Model file for the job. Use its own axes, mm. A direction names the side the tool comes from. Coordinates: 2 decimals unless noted, no trailing zeros. Loops run counter-clockwise (first coordinate to the right, second up) from the corner with the lowest first, then second, coordinate; pieces in that order, holes last. Notation, with made-up numbers: M 46.5,26 L 85.5,26 A25 ccw 85.5,63 Z; hole C 77,-11.75 d1. An arc over 180 degrees is marked long. Write item = value, one per line. Start each with the question number.
Autodesk Inventor part; units mm, degrees
ref_plane "YZ Plane" through (0, 0, 0) normal (1, 0, 0) x (0, 1, 0)
ref_plane "XZ Plane" through (0, 0, 0) normal (0, 1, 0) x (-1, 0, 0)
ref_plane "XY Plane" through (0, 0, 0) normal (0, 0, 1) x (1, 0, 0)
sketch "Sketch1" plane through (0, 0, 0) normal (0, 1, 0) x (-1, 0, 0)
  line L0 (0, 0) -> (108.6, 0)
  line L1 (108.6, 0) -> (108.6, -110.4)
  line L2 (108.6, -110.4) -> (0, -110.4)
  line L3 (0, -110.4) -> (0, 0)
  circle A0 centre (12.3, -77.7) radius 6.5
  circle A1 centre (57.3, -77.7) radius 12
  dimension "d0" = 108.6
  dimension "d1" = 110.4
  dimension "d2" = 13
  dimension "altura_hoyo" = 12.3
  dimension "d5" = 32.7
  dimension "d6" = 24
  dimension "d7" = 45
extrude "Extrusion1" add sketch "Sketch1" along normal blind 27
sketch "Sketch2" plane through (0, 27, 0) normal (0, 1, 0) x (1, 0, 0)
  line L0 (0, 110.4) -> (-108.6, 110.4) construction
  line L1 (0, 0) -> (0, -195.629)
  line L2 (0, -195.629) -> (0, -201.129)
  line L3 (0, -201.129) -> (-188.5967, -306.4251)
  line L4 (-24.6, 0) -> (-24.6, -190.129)
  line L5 (-188.5967, -281.6906) -> (-24.6, -190.129)
  line L6 (-188.5967, -306.4251) -> (-188.5967, -281.6906)
  circle A0 centre (-12.3, -195.629) radius 7.8
  circle A1 centre (-12.3, 77.7) radius 6.5 construction
  line L7 (-108.6, 0) -> (0, 0)
  line L8 (0, 0) -> (-24.6, 0)
  line L9 (-12.3, -195.629) -> (-149.732, -272.3592) construction
  line L10 (0, -201.129) -> (-12.3, -195.629) construction
  line L11 (-42.6296, -182.067) -> (-12.3, -195.629) construction
  circle A2 centre (-149.732, -272.3592) radius 7.8
  dimension "d10" = 306.029
  dimension "d11" = 5.5
  dimension "d12" = 119.175
  dimension "Ancho_marco" = 24.6
  dimension "d18" = 15.6
  dimension "d21" = 216
  dimension "d26" = 12.3
  dimension "d_entre_ejes" = 157.401
  dimension "d28" = 15.6
  dimension "d31" = 195.629
  dimension "d32" = 273.329
extrude "Extrusion2" add sketch "Sketch2" against normal blind 27 contours L1 L2 L3 L6 L5 L4 L7 | A2
fillet "Fillet1" radius 10 2 edges at (-24.6, 13.5, 190.129) (0, 13.5, 201.129)
sketch "Sketch3" plane through (0, 27, 0) normal (0, 1, 0) x (1, 0, 0)
  line L0 (-188.5967, -281.6906) -> (-188.5967, -306.4251)
  line L1 (-188.5967, -306.4251) -> (-200.2967, -306.4251)
  line L2 (-200.2967, -306.4251) -> (-200.2967, -288.2229)
  line L3 (-188.5967, -306.4251) -> (-188.5967, -281.6906)
  line L4 (-188.5967, -281.6906) -> (-200.2967, -288.2229)
  line L5 (-29.7252, -192.9905) -> (-188.5967, -281.6906)
  point P0 (0, 0)
  dimension "d23" = 11.7
extrude "Extrusion3" add sketch "Sketch3" against normal blind 27
extrude "Extrusion4" cut sketch "Sketch2" against normal blind 27 contours A2
equation "\"d11\" = 0.5 * D_eje"
equation "\"d18\" = d28"
properties part number "Marco_triciclo" material "Aluminum 6061"
Item 1: Probe L1, parallel to Z at x = -57.3, y = 9; L2, parallel to Z at x = -14.5, y = 3.25; L3, parallel to Z at x = -77, y = 22. List the from-to ranges inside material, lowest first.
Item 2: Cut at C-C (y = 16.25). Give the cut face in (x, z), plus the area to 3 significant figures.
Item 3: Pull direction X, two halves, no side cores. Call faces 4 (the flat face through (-95.577, 13.689, 254.491)), 5 (the cylindrical face through (-25.94, 13.31, 189.26)), 6 (the cylindrical face through (-68.746, 13.311, -81.304)): +X half, -X half, draft (parallel to the pull), parting line (faces both ways), or undercut.
Item 4: 3-axis set-ups, long thin cutter, end or side, ignore diameter. For faces 1 (the flat face through (-19, 0, 35)), 2 (the flat face through (-24.6, 14, 91)), 3 (the flat face through (-108.6, 13, -54)): which of +Z, -Z, +X, -X, +Y, -Y reach the whole face in a straight line?
Item 5: Cut at D-D (z = -11.5). Give the cut face in (x, y), plus the area to 3 significant figures.
Item 6: Pin check, flat tips, straight feed: pin 1 Ø8 at (y, z) = (16, 108.5) entering from -X; pin 2 Ø13.5 at (y, z) = (11.5, -29.5) entering from -X. Stop position of each tip, or through.
Item 7: Cut at A-A (z = -77.7). Give the cut face in (x, y), plus the area to 3 significant figures.
Item 8: Cut at B-B (x = -57.3). Give the cut face in (y, z).
Reported:
q1.L1 = -110.4 to -89.7, -65.7 to 0, 208.39 to 233.12
q1.L2 = -110.4 to -83.82, -71.58 to 188.15, 203.11 to 209.22
q1.L3 = -110.4 to 0, 219.38 to 244.12
q2.outline = M -200.3,288.22 L -188.6,281.69 L -29.73,192.99 A10 cw -24.6,184.26 L -24.6,0 L -108.6,0 L -108.6,-110.4 L 0,-110.4 L 0,195.26 A10 ccw -5.13,203.99 L -188.6,306.43 L -200.3,306.43 Z; hole C -149.73,272.36 d15.6; hole C -57.3,-77.7 d24; hole C -12.3,195.63 d15.6; hole C -12.3,-77.7 d13
q2.area = 20,400 mm^2
q3.face_4 = +X half
q3.face_5 = -X half
q3.face_6 = undercut
q4.face_1 = +Z, -Z, +X, -X, -Y
q4.face_2 = -X, +Y, -Y
q4.face_3 = -Z, -X, +Y, -Y
q5.outline = M -108.6,0 L 0,0 L 0,27 L -108.6,27 Z
q5.area = 2,930 mm^2
q6.pin_1 = -24.6
q6.pin_2 = -108.6
q7.outline = M -108.6,0 L -69.3,0 L -69.3,27 L -108.6,27 Z; M -45.3,0 L -18.8,0 L -18.8,27 L -45.3,27 Z; M -5.8,0 L 0,0 L 0,27 L -5.8,27 Z
q7.area = 1,930 mm^2
q8.outline = M 0,-110.4 L 27,-110.4 L 27,-89.7 L 0,-89.7 Z; M 0,-65.7 L 27,-65.7 L 27,0 L 0,0 Z; M 0,208.39 L 27,208.39 L 27,233.12 L 0,233.12 Z
